from build123d import *

# Parameters (mm, degrees)
SKETCH1_R           = 42
BOSS_EXTRUDE1_DEPTH = 1.5


with BuildPart() as part:
    # Sketch1 → Boss-Extrude1 (new, symmetric)
    with BuildSketch(Plane(origin=(0, 0, 0), x_dir=(0, 0, -1), z_dir=(1, 0, 0))):
        Circle(SKETCH1_R)
        with BuildLine():
            Line((-1.5, 38.97114317), (-1.5, 31.964824417))
            ThreePointArc((-1.5, 31.964824417), (-22.627416998, 22.627416998), (-31.964824417, 1.5))
            Line((-31.964824417, 1.5), (-38.97114317, 1.5))
            ThreePointArc((-38.97114317, 1.5), (-27.577164466, 27.577164466), (-1.5, 38.97114317))
        make_face(mode=Mode.SUBTRACT)
        with BuildLine():
            Line((1.5, 38.97114317), (1.5, 31.964824417))
            ThreePointArc((1.5, 31.964824417), (22.627416998, 22.627416998), (31.964824417, 1.5))
            Line((31.964824417, 1.5), (38.97114317, 1.5))
            ThreePointArc((38.97114317, 1.5), (27.577164466, 27.577164466), (1.5, 38.97114317))
        make_face(mode=Mode.SUBTRACT)
        with BuildLine():
            Line((38.97114317, -1.5), (31.964824417, -1.5))
            ThreePointArc((31.964824417, -1.5), (22.627416998, -22.627416998), (1.5, -31.964824417))
            Line((1.5, -31.964824417), (1.5, -38.97114317))
            ThreePointArc((1.5, -38.97114317), (27.577164466, -27.577164466), (38.97114317, -1.5))
        make_face(mode=Mode.SUBTRACT)
        with BuildLine():
            Line((-1.5, -38.97114317), (-1.5, -31.964824417))
            ThreePointArc((-1.5, -31.964824417), (-22.627416998, -22.627416998), (-31.964824417, -1.5))
            Line((-31.964824417, -1.5), (-38.97114317, -1.5))
            ThreePointArc((-38.97114317, -1.5), (-27.577164466, -27.577164466), (-1.5, -38.97114317))
        make_face(mode=Mode.SUBTRACT)
        with BuildLine():
            Line((-28.961180915, 1.5), (-21.948804068, 1.5))
            ThreePointArc((-21.948804068, 1.5), (-15.556349186, 15.556349186), (-1.5, 21.948804068))
            Line((-1.5, 21.948804068), (-1.5, 28.961180915))
            ThreePointArc((-1.5, 28.961180915), (-20.506096654, 20.506096654), (-28.961180915, 1.5))
        make_face(mode=Mode.SUBTRACT)
        with BuildLine():
            Line((-18.940696925, 1.5), (-11.9058809, 1.5))
            ThreePointArc((-11.9058809, 1.5), (-8.485281374, 8.485281374), (-1.5, 11.9058809))
            Line((-1.5, 11.9058809), (-1.5, 18.940696925))
            ThreePointArc((-1.5, 18.940696925), (-13.435028843, 13.435028843), (-18.940696925, 1.5))
        make_face(mode=Mode.SUBTRACT)
        with BuildLine():
            Line((-8.874119675, 1.5), (-1.5, 1.5))
            Line((-1.5, 1.5), (-1.5, 8.874119675))
            ThreePointArc((-1.5, 8.874119675), (-6.363961031, 6.363961031), (-8.874119675, 1.5))
        make_face(mode=Mode.SUBTRACT)
        with BuildLine():
            Line((-28.961180915, -1.5), (-21.948804068, -1.5))
            ThreePointArc((-21.948804068, -1.5), (-15.556349186, -15.556349186), (-1.5, -21.948804068))
            Line((-1.5, -21.948804068), (-1.5, -28.961180915))
            ThreePointArc((-1.5, -28.961180915), (-20.506096654, -20.506096654), (-28.961180915, -1.5))
        make_face(mode=Mode.SUBTRACT)
        with BuildLine():
            Line((-18.940696925, -1.5), (-11.9058809, -1.5))
            ThreePointArc((-11.9058809, -1.5), (-8.485281374, -8.485281374), (-1.5, -11.9058809))
            Line((-1.5, -11.9058809), (-1.5, -18.940696925))
            ThreePointArc((-1.5, -18.940696925), (-13.435028843, -13.435028843), (-18.940696925, -1.5))
        make_face(mode=Mode.SUBTRACT)
        with BuildLine():
            Line((-8.874119675, -1.5), (-1.5, -1.5))
            Line((-1.5, -1.5), (-1.5, -8.874119675))
            ThreePointArc((-1.5, -8.874119675), (-6.363961031, -6.363961031), (-8.874119675, -1.5))
        make_face(mode=Mode.SUBTRACT)
        with BuildLine():
            Line((1.5, -28.961180915), (1.5, -21.948804068))
            ThreePointArc((1.5, -21.948804068), (15.556349186, -15.556349186), (21.948804068, -1.5))
            Line((21.948804068, -1.5), (28.961180915, -1.5))
            ThreePointArc((28.961180915, -1.5), (20.506096654, -20.506096654), (1.5, -28.961180915))
        make_face(mode=Mode.SUBTRACT)
        with BuildLine():
            Line((1.5, -18.940696925), (1.5, -11.9058809))
            ThreePointArc((1.5, -11.9058809), (8.485281374, -8.485281374), (11.9058809, -1.5))
            Line((11.9058809, -1.5), (18.940696925, -1.5))
            ThreePointArc((18.940696925, -1.5), (13.435028843, -13.435028843), (1.5, -18.940696925))
        make_face(mode=Mode.SUBTRACT)
        with BuildLine():
            Line((1.5, -8.874119675), (1.5, -1.5))
            Line((1.5, -1.5), (8.874119675, -1.5))
            ThreePointArc((8.874119675, -1.5), (6.363961031, -6.363961031), (1.5, -8.874119675))
        make_face(mode=Mode.SUBTRACT)
        with BuildLine():
            Line((8.874119675, 1.5), (1.5, 1.5))
            Line((1.5, 1.5), (1.5, 8.874119675))
            ThreePointArc((1.5, 8.874119675), (6.363961031, 6.363961031), (8.874119675, 1.5))
        make_face(mode=Mode.SUBTRACT)
        with BuildLine():
            Line((18.940696925, 1.5), (11.9058809, 1.5))
            ThreePointArc((11.9058809, 1.5), (8.485281374, 8.485281374), (1.5, 11.9058809))
            Line((1.5, 11.9058809), (1.5, 18.940696925))
            ThreePointArc((1.5, 18.940696925), (13.435028843, 13.435028843), (18.940696925, 1.5))
        make_face(mode=Mode.SUBTRACT)
        with BuildLine():
            Line((28.961180915, 1.5), (21.948804068, 1.5))
            ThreePointArc((21.948804068, 1.5), (15.556349186, 15.556349186), (1.5, 21.948804068))
            Line((1.5, 21.948804068), (1.5, 28.961180915))
            ThreePointArc((1.5, 28.961180915), (20.506096654, 20.506096654), (28.961180915, 1.5))
        make_face(mode=Mode.SUBTRACT)
    extrude(amount=BOSS_EXTRUDE1_DEPTH, both=True)


solid = part.part
Verification items for the finished model (mm, model axes). Give positions to 0.01 mm unless a question says otherwise; leave off trailing zeros. Write each loop counter-clockwise with the first axis right and the second up, starting at its lowest first coordinate (ties: lowest second). Pieces come first, ordered by that corner, then holes. Notation, with made-up numbers: (-29.5, 11) - (-8.5, 11) arc R15 cw to (-8.5, 39) - close; hole circle Ø11 at (48, 70.25). An arc over 180 degrees is marked (long way). Answer as CSV lines item,"result". Start each with the question number.
1. Depth check by flat-ended pin: pin 1 (0.9 mm diameter, centred on x = -0.5, z = -36.5, fed in from -Y); pin 2 (1.5 mm diameter, centred on x = 0, z = 4.5, fed in from +Y); pin 3 (1.5 mm diameter, centred on x = -0.5, z = -27, fed in from -Y). Enter the tip coordinate at first touch or a pass-through.
2. Sectioned sample at A-A (z = -13). Record the boundary of the cut face in (x, y).
3. Sectioned sample at D-D (z = 30.5). Record the boundary of the cut face in (x, y), then the cut area to 3 significant figures.
4. Thickness scan on line 1 (Z direction, x = 0.4, y = 34); line 2 (Z direction, x = -0.2, y = 22.5); line 3 (Z direction, x = -0.25, y = 35). Record the ranges inside material, lowest first.
5. Sectioned sample at B-B (y = 14). Record the boundary of the cut face in (x, z), then the cut area to 3 significant figures.
6. Draft check along Y on faces 1 (the face through (0.02, 12.62, -40.06)), 2 (the face through (0, -26, -1.5)), 3 (the face through (0, -36, 1.5)), 4 (the face through (-1.5, 1, 1)). Enter one of: pulls with the +Y half, pulls with the -Y half, needs draft (parallel to the pull), parting line crosses it, or undercut.
7. Sectioned sample at C-C (x = -1.05). Count the separate pieces of the cut face and the enclosed holes in it, then the cut area to 3 significant figures.
Derived:
1,pin 1,"y = -21.55"
1,pin 2,"y = 41.83"
1,pin 3,"y = -32.79"
2,outline,"(-1.5, -39.94) - (1.5, -39.94) - (1.5, -36.77) - (-1.5, -36.77) - close; (-1.5, -29.24) - (1.5, -29.24) - (1.5, -25.92) - (-1.5, -25.92) - close; (-1.5, -17.75) - (1.5, -17.75) - (1.5, -13.86) - (-1.5, -13.86) - close; (-1.5, -1.5) - (1.5, -1.5) - (1.5, 1.5) - (-1.5, 1.5) - close; (-1.5, 13.86) - (1.5, 13.86) - (1.5, 17.75) - (-1.5, 17.75) - close; (-1.5, 25.92) - (1.5, 25.92) - (1.5, 29.24) - (-1.5, 29.24) - close; (-1.5, 36.77) - (1.5, 36.77) - (1.5, 39.94) - (-1.5, 39.94) - close"
3,outline,"(-1.5, -28.87) - (1.5, -28.87) - (1.5, -24.31) - (-1.5, -24.31) - close; (-1.5, -9.68) - (1.5, -9.68) - (1.5, 9.68) - (-1.5, 9.68) - close; (-1.5, 24.31) - (1.5, 24.31) - (1.5, 28.87) - (-1.5, 28.87) - close"
3,area,"85.5 mm²"
4,line 1,"-24.66 to -19.1, -1.5 to 1.5, 19.1 to 24.66"
4,line 2,"-35.46 to -31.86, -22.75 to -18.3, -1.5 to 1.5, 18.3 to 22.75, 31.86 to 35.46"
4,line 3,"-23.22 to -17.2, -1.5 to 1.5, 17.2 to 23.22"
5,outline,"(-1.5, -39.6) - (1.5, -39.6) - (1.5, -36.4) - (-1.5, -36.4) - close; (-1.5, -28.77) - (1.5, -28.77) - (1.5, -25.4) - (-1.5, -25.4) - close; (-1.5, -16.97) - (1.5, -16.97) - (1.5, -12.85) - (-1.5, -12.85) - close; (-1.5, -1.5) - (1.5, -1.5) - (1.5, 1.5) - (-1.5, 1.5) - close; (-1.5, 12.85) - (1.5, 12.85) - (1.5, 16.97) - (-1.5, 16.97) - close; (-1.5, 25.4) - (1.5, 25.4) - (1.5, 28.77) - (-1.5, 28.77) - close; (-1.5, 36.4) - (1.5, 36.4) - (1.5, 39.6) - (-1.5, 39.6) - close"
5,area,"73.2 mm²"
6,face 1,"parting line crosses it"
6,face 2,"undercut"
6,face 3,"undercut"
6,face 4,"needs draft"
7,separate pieces,"1"
7,enclosed holes,"16"
7,area,"2,270 mm²"
